from build123d import *

# Parameters (mm, degrees)
SKETCH1_R           = 2.5
SKETCH1_W           = 350
SKETCH1_H           = 475
BOSS_EXTRUDE1_DEPTH = 12.5
BOSS_EXTRUDE2_START = -15
SKETCH2_R           = 2.5
BOSS_EXTRUDE2_DEPTH = 15
FILLET1_R           = 10
FILLET2_R           = 30
FILLET3_R           = 10


with BuildPart() as part:
    # Sketch1 → Boss-Extrude1 (new, symmetric)
    with BuildSketch(Plane(origin=(0, 0, 0), x_dir=(0, 0, -1), z_dir=(1, 0, 0))):
        Polygon((-175, -337.5), (-225, -337.5), (-225, 337.5), (225, 337.5), (225, -337.5), (175, -337.5), (175, -287.5), (-175, -287.5), align=None)
        with Locations((-150, 330)):
            Circle(SKETCH1_R, mode=Mode.SUBTRACT)
        with Locations((-110, 330)):
            Circle(SKETCH1_R, mode=Mode.SUBTRACT)
        with Locations((-130, 315)):
            Circle(SKETCH1_R, mode=Mode.SUBTRACT)
        with Locations(Location((110, 330, 0), (0, 0, 180))):
            Circle(SKETCH1_R, mode=Mode.SUBTRACT)
        with Locations(Location((150, 330, 0), (0, 0, 180))):
            Circle(SKETCH1_R, mode=Mode.SUBTRACT)
        with Locations(Location((130, 315, 0), (0, 0, 180))):
            Circle(SKETCH1_R, mode=Mode.SUBTRACT)
        Rectangle(SKETCH1_W, SKETCH1_H, mode=Mode.SUBTRACT)
    extrude(amount=BOSS_EXTRUDE1_DEPTH, both=True)

    # Sketch2 → Boss-Extrude2 (add)
    with BuildSketch(Plane(origin=(12.5, 0, 0), x_dir=(0, 0, -1), z_dir=(1, 0, 0)).offset(BOSS_EXTRUDE2_START)):
        with Locations((-110, 330)):
            Circle(SKETCH2_R)
        with Locations((-130, 315)):
            Circle(SKETCH2_R)
        with Locations((-150, 330)):
            Circle(SKETCH2_R)
        with Locations(Location((150, 330, 0), (0, 0, 180))):
            Circle(SKETCH2_R)
        with Locations(Location((130, 315, 0), (0, 0, 180))):
            Circle(SKETCH2_R)
        with Locations(Location((110, 330, 0), (0, 0, 180))):
            Circle(SKETCH2_R)
    extrude(amount=BOSS_EXTRUDE2_DEPTH)

    # Fillet1
    fillet1_edges = [part.edges().sort_by_distance(p)[0] for p in [
        (0, -287.5, -175),
        (0, -287.5, 175),
    ]]
    fillet(fillet1_edges, radius=FILLET1_R)

    # Fillet2
    fillet2_edges = [part.edges().sort_by_distance(p)[0] for p in [
        (0, 237.5, 175),
        (0, -237.5, 175),
        (0, -237.5, -175),
        (0, 237.5, -175),
    ]]
    fillet(fillet2_edges, radius=FILLET2_R)

    # Fillet3
    fillet3_edges = [part.edges().sort_by_distance(p)[0] for p in [
        (0, 337.5, 225),
        (0, 337.5, -225),
    ]]
    fillet(fillet3_edges, radius=FILLET3_R)


solid = part.part
Check sheet for the modelled part. Datum: model origin and axes. Units: mm. A direction names the side the tool comes from. Coordinates: 2 decimals unless noted, no trailing zeros. Write each loop counter-clockwise with the first axis right and the second up, starting at its lowest first coordinate (ties: lowest second). Pieces come first, ordered by that corner, then holes. Notation, with made-up numbers: M 4,21.25 L 36,21.25 A8 ccw 36,36.25 Z; hole C 63.5,59 d4. An arc over 180 degrees is marked long. Answer as CSV lines item,"result".
Q1. Cross-section at A-A (x = 5). Record the boundary of the cut face in (y, z).
Check result:
outline,"M -337.5,-225 L 327.5,-225 A10 ccw 337.5,-215 L 337.5,215 A10 ccw 327.5,225 L -337.5,225 L -337.5,175 L -297.5,175 A10 cw -287.5,165 L -287.5,-165 A10 cw -297.5,-175 L -337.5,-175 Z; hole M -237.5,-145 A30 ccw -207.5,-175 L 207.5,-175 A30 ccw 237.5,-145 L 237.5,145 A30 ccw 207.5,175 L -207.5,175 A30 ccw -237.5,145 Z"
Q2. Material ranges on probe 1 along Y at (x, z) = (-9.5, 110); probe 2 along Y at (x, z) = (-6, 130); probe 3 along Z at (x, y) = (-5.5, 315), recorded low to high. Write a range as from..to.
Check result:
probe 1,"-287.5..-237.5, 237.5..327.5, 332.5..337.5"
probe 2,"-287.5..-237.5, 237.5..312.5, 317.5..337.5"
probe 3,"-225..-132.5, -127.5..127.5, 132.5..225"
Q3. Go/stop test with flat-tipped pins: pin 1 (4 mm diameter, centred on x = -2.5, z = 65, fed in from -Y); pin 2 (2.5 mm diameter, centred on y = 330, z = 110, fed in from -X); pin 3 (2.5 mm diameter, centred on y = 329, z = -111, fed in from -X). Record where each tip stops, or that it passes through.
Check result:
pin 1,"y = -287.5"
pin 2,"x = -2.5"
pin 3,"x = -12.5"
Q4. Cross-section at C-C (z = 31). Record the boundary of the cut face in (x, y).
Check result:
outline,"M -12.5,-287.5 L 12.5,-287.5 L 12.5,-237.5 L -12.5,-237.5 Z; M -12.5,237.5 L 12.5,237.5 L 12.5,337.5 L -12.5,337.5 Z"
Q5. Set-up check for faces 4 (the face through (-0.175, -228.479, 166.445)), 5 (the face through (0, -318, -175)), 6 (the face through (0, 0, -225)): record each of +Z, -Z, +X, -X, +Y, -Y from which the full face is reachable in a straight line by a thin tool's end or side.
Check result:
face 4,"+X, -X"
face 5,"+X, -X, -Y"
face 6,"-Z, +X, -X, +Y, -Y"
Q6. Mould release check, pull along Y, two halves, no side actions. Record for faces 1 (the face through (0, -287.5, -2)), 2 (the face through (0, -317, 175)), 3 (the face through (0.175, -228.479, -166.445)): released by +Y, released by -Y, zero draft, split by the parting line, or undercut.
Check result:
face 1,"released by -Y"
face 2,"zero draft"
face 3,"undercut"
Q7. Cross-section at B-B (y = 89). Record the boundary of the cut face in (x, z), then the cut area to 3 significant figures.
Check result:
outline,"M -12.5,-225 L 12.5,-225 L 12.5,-175 L -12.5,-175 Z; M -12.5,175 L 12.5,175 L 12.5,225 L -12.5,225 Z"
area,"2,500 mm^2"
